Design review of the part built by this model. Coordinates are the model's own, in mm. A direction names the side the tool comes from. Coordinates: 2 decimals unless noted, no trailing zeros. Loops run counter-clockwise (first coordinate to the right, second up) from the corner with the lowest first, then second, coordinate; pieces in that order, holes last. Notation, with made-up numbers: M -3.5,40.25 L 40.5,40.25 A10 ccw 40.5,52.25 Z; hole C -4,16 d6. An arc over 180 degrees is marked long. Write item = value, one per line. Start each with the question number.
```python
from build123d import *

# Parameters (mm, degrees)
F1_DEPTH = 12


with BuildPart() as f1:
    # F0 (on Front) → F1 (new body)
    with BuildSketch(Plane.XZ):
        with BuildLine():
            Line((-180, -217.421149), (-180, -240))
            Line((-180, -240), (-112.5, -240))
            ThreePointArc((-112.5, -240), (-81.643279, -162.600872), (-6, -127.660114))
            Line((-6, -127.660114), (-6, 52.5))
            ThreePointArc((-6, 52.5), (0, 58.5), (6, 52.5))
            Line((6, 52.5), (6, -127.660114))
            ThreePointArc((6, -127.660114), (81.643279, -162.600872), (112.5, -240))
            Line((112.5, -240), (180, -240))
            Line((180, -240), (180, -217.421149))
            ThreePointArc((180, -217.421149), (171.168592, -166.711894), (145.714286, -121.97376))
            ThreePointArc((145.714286, -121.97376), (100, 5.289425), (145.714286, 132.552611))
            ThreePointArc((145.714286, 132.552611), (171.168592, 177.290745), (180, 228))
            Line((180, 228), (180, 240))
            Line((180, 240), (130, 240))
            Line((130, 240), (130, 228))
            Line((130, 228), (130, 220))
            ThreePointArc((130, 220), (123, 213), (116, 220))
            Line((116, 220), (116, 226))
            ThreePointArc((116, 226), (115.414214, 227.414214), (114, 228))
            Line((114, 228), (-113.99243, 228))
            ThreePointArc((-113.99243, 228), (-115.405751, 227.415105), (-115.992428, 226.002523))
            Line((-115.992428, 226.002523), (-116, 220))
            ThreePointArc((-116, 220), (-123, 213), (-130, 220))
            Line((-130, 220), (-130, 228))
            Line((-130, 228), (-130, 240))
            Line((-130, 240), (-180, 240))
            Line((-180, 240), (-180, 228))
            ThreePointArc((-180, 228), (-171.168592, 177.290745), (-145.714286, 132.552611))
            ThreePointArc((-145.714286, 132.552611), (-100, 5.289425), (-145.714286, -121.97376))
            ThreePointArc((-145.714286, -121.97376), (-171.168592, -166.711894), (-180, -217.421149))
        make_face()
    extrude(amount=F1_DEPTH)


solid = f1.part
```
(1) Tool access review of faces 1 (the flat face through (-6, -6, -39)), 2 (the cylindrical face through (-170.92, -5.92, -166.03)), 3 (the flat face through (-130, -6, 230)), 4 (the cylindrical face through (170.922, -5.916, 176.61)), 5 (the flat face through (-43, -12, 3)): name each direction out of +Z, -Z, +X, -X, +Y, -Y from which nothing blocks a thin tool from reaching the whole face with its end or side.
(2) Take a section at C-C (y = -9.25). State the section outline as (x, z) points.
(3) Mouldability with a two-part tool opening along Z and no side actions: class faces 6 (the cylindrical face through (171.41, -5.92, -167.39)), 7 (the flat face through (180, -6, 234)), 8 (the flat face through (155, -6, 240)) as +Z half, -Z half, draft (parallel to the pull), parting line (faces both ways), or undercut.
(4) Take a section at D-D (x = 0). State the section outline as (y, z) points.
(5) To check wall thickness, follow L1, parallel to X at y = -8.75, z = 5.5; L2, parallel to Z at x = -165, y = -9.5; L3, parallel to X at y = -4.75, z = -205. State the ranges of each line that lie inside material, in increasing order.
(6) Take a section at B-B (z = -22.5). State the section outline as (x, y) points.
(7) Take a section at A-A (x = -123). State the section outline as (y, z) points.
(8) Insertion check: pin 1 (6 mm diameter, centred on x = -12, y = -5, fed in from +Z); pin 2 (3.5 mm diameter, centred on y = -3.5, z = -34, fed in from +X); pin 3 (5 mm diameter, centred on y = -4.5, z = 222, fed in from +X). Each pin has a flat end and moves straight along its axis. Give the tip position at first contact, or say it passes through.
Results list:
q1.face_1 = -Z, +Y, -Y
q1.face_2 = -X, +Y, -Y
q1.face_3 = +Z, +Y, -Y
q1.face_4 = +X, +Y, -Y
q1.face_5 = +Z, -Z, +X, -X, -Y
q2.outline = M -180,-240 L -112.5,-240 A112.5 cw -6,-127.66 L -6,52.5 A6 cw 6,52.5 L 6,-127.66 A112.5 cw 112.5,-240 L 180,-240 L 180,-217.42 A150 ccw 145.71,-121.97 A200 cw 145.71,132.55 A150 ccw 180,228 L 180,240 L 130,240 L 130,220 A7 cw 116,220 L 116,226 A2 ccw 114,228 L -113.99,228 A2 ccw -115.99,226 L -116,220 A7 cw -130,220 L -130,240 L -180,240 L -180,228 A150 ccw -145.71,132.55 A200 cw -145.71,-121.97 A150 ccw -180,-217.42 Z
q3.face_6 = undercut
q3.face_7 = draft
q3.face_8 = +Z half
q4.outline = M -12,58.5 L 0,58.5 L 0,228 L -12,228 Z
q5.L1 = -100 to -6, 6 to 100
q5.L2 = -240 to -152.04, 162.62 to 240
q5.L3 = -179.48 to -106.92, 106.92 to 179.48
q6.outline = M -101.94,-12 L -6,-12 L -6,0 L -101.94,0 Z; M 6,-12 L 101.94,-12 L 101.94,0 L 6,0 Z
q7.outline = M -12,-240 L 0,-240 L 0,-87.83 L -12,-87.83 Z; M -12,98.41 L 0,98.41 L 0,213 L -12,213 Z
q8.pin_1 = 228
q8.pin_2 = 104.26
q8.pin_3 = 179.96
